from build123d import *

# Parameters (mm, degrees)
SKETCH1_W           = 40
SKETCH1_H           = 40
BOSS_EXTRUDE1_DEPTH = 60
SKETCH3_W           = 10
SKETCH3_H           = 40
CUT_EXTRUDE1_DEPTH  = 60
CUT_EXTRUDE2_DEPTH  = 30
SKETCH5_W           = 10
SKETCH5_H           = 60
CUT_EXTRUDE3_DEPTH  = 30
SKETCH6_W           = 20
SKETCH6_H           = 30
CUT_EXTRUDE4_DEPTH  = 10
SKETCH7_W           = 20
SKETCH7_H           = 15
CUT_EXTRUDE5_DEPTH  = 20


with BuildPart() as part:
    # Sketch1 → Boss-Extrude1 (new body)
    with BuildSketch(Plane.XY):
        with Locations((20, 20)):
            Rectangle(SKETCH1_W, SKETCH1_H)
    extrude(amount=BOSS_EXTRUDE1_DEPTH)

    # Sketch3 → Cut-Extrude1 (cut)
    with BuildSketch(Plane(origin=(0, 40, 0), x_dir=(1, 0, 0), z_dir=(0, 1, 0))):
        with Locations((5, -30)):
            Rectangle(SKETCH3_W, SKETCH3_H)
    extrude(amount=-CUT_EXTRUDE1_DEPTH, mode=Mode.SUBTRACT)

    # Sketch4 → Cut-Extrude2 (cut)
    with BuildSketch(Plane(origin=(0, 40, 0), x_dir=(1, 0, 0), z_dir=(0, 1, 0))):
        Polygon((10, -10), (10, -60), (20, -60), (20, -10), (20, 0), (10, 0), align=None)
    extrude(amount=-CUT_EXTRUDE2_DEPTH, mode=Mode.SUBTRACT)

    # Sketch5 → Cut-Extrude3 (cut)
    with BuildSketch(Plane(origin=(0, 40, 0), x_dir=(1, 0, 0), z_dir=(0, 1, 0))):
        with Locations((5, -30)):
            Rectangle(SKETCH5_W, SKETCH5_H)
    extrude(amount=-CUT_EXTRUDE3_DEPTH, mode=Mode.SUBTRACT)

    # Sketch6 → Cut-Extrude4 (cut)
    with BuildSketch(Plane(origin=(0, 40, 0), x_dir=(1, 0, 0), z_dir=(0, 1, 0))):
        with Locations((30, -15)):
            Rectangle(SKETCH6_W, SKETCH6_H)
    extrude(amount=-CUT_EXTRUDE4_DEPTH, mode=Mode.SUBTRACT)

    # Sketch7 → Cut-Extrude5 (cut)
    with BuildSketch(Plane(origin=(0, 40, 0), x_dir=(1, 0, 0), z_dir=(0, 1, 0))):
        with Locations((30, -52.5)):
            Rectangle(SKETCH7_W, SKETCH7_H)
    extrude(amount=-CUT_EXTRUDE5_DEPTH, mode=Mode.SUBTRACT)


solid = part.part
Could you check a few things on this model? Use its own coordinates, in mm. A direction names the side the tool comes from. Give positions to 0.01 mm unless a question says otherwise; leave off trailing zeros. Order: outer loops, then holes, each group sorted by start corner. A loop starts at its lowest first (then second) coordinate and runs counter-clockwise, first axis right, second up.
1. For faces 1 (the flat face through (10, 5, 30)), 2 (the flat face through (20, 22, 30)), 3 (the flat face through (30, 30, 15)), 4 (the flat face through (30, 30, 45)), which set-ups out of +Z, -Z, +X, -X, +Y, -Y let a thin tool reach every point of the face, with its end or its side?
2. Suppose I cut it at D-D (y = 34). List the corners of the cut face in (x, z) for me.
3. Suppose I cut it at A-A (x = 21). List the corners of the cut face in (y, z) for me, plus the area to 3 significant figures.
4. Suppose I cut it at B-B (y = 8.5). List the corners of the cut face in (x, z) for me, plus the area to 3 significant figures.
5. Suppose I cut it at C-C (z = 41). List the corners of the cut face in (x, y) for me.
6. Will these pins go through, and if not, where does the flat tip stop? P1, Ø1.5, axis at x = 14, y = 9, coming from the -Z side; P2, Ø24, axis at y = 28, z = 34.5, coming from the -X side; P3, Ø11, axis at y = 7.5, z = 24, coming from the -X side; P4, Ø10, axis at x = 6, z = 44.5, coming from the +Y side.
7. We'd pull the mould along Z, two halves only. Please class faces 5 (the flat face through (24, 8, 60)), 6 (the flat face through (24, 0, 30)), 7 (the flat face through (5, 5, 10)): pulls with the +Z half, pulls with the -Z half, needs draft (parallel to the pull), parting line crosses it, or undercut.
8. I need wall thicknesses on L1, parallel to X at y = 9, z = 22; L2, parallel to Y at x = 18, z = 8; L3, parallel to Y at x = 35.5, z = 18.5. Which ranges of each line are inside material? Lowest first, please.
Solved:
1. face 1: -X, +Y, -Y
1. face 2: +Z, -Z, -X, +Y
1. face 3: -Z, +X, -X, +Y
1. face 4: +Z, +X, -X, +Y
2. outline: (20, 30) - (40, 30) - (40, 45) - (20, 45) - close
3. outline: (0, 0) - (30, 0) - (30, 30) - (40, 30) - (40, 45) - (20, 45) - (20, 60) - (0, 60) - close
3. area: 1,800 mm2
4. outline: (0, 0) - (40, 0) - (40, 60) - (0, 60) - (0, 50) - (10, 50) - (10, 10) - (0, 10) - close
4. area: 2,000 mm2
5. outline: (10, 0) - (40, 0) - (40, 40) - (20, 40) - (20, 10) - (10, 10) - close
6. P1: stops at z = 0
6. P2: stops at x = 20
6. P3: stops at x = 10
6. P4: stops at y = 10
7. face 5: pulls with the +Z half
7. face 6: needs draft
7. face 7: undercut
8. L1: x = 10 to 40
8. L2: y = 0 to 10
8. L3: y = 0 to 30
